Build history of the part. All positions in model axes, mm. A direction names the side the tool comes from. Coordinates: 2 decimals unless noted, no trailing zeros. One line per item, written item: value.
```python
from build123d import *

# Parameters (mm, degrees)
EXTRUDE_1_DEPTH          = 1
SKETCH_2_R               = 5
CUT_EXTRUDE_2_DEPTH      = 302.498287555
SKETCH_7_W               = 10
SKETCH_7_H               = 4
EXTRUDE_2_DEPTH          = 10
CUT_EXTRUDE_3_DEPTH      = 303.724763765
CUT_EXTRUDE_3_DEPTH_BACK = 303.724763765
SKETCH_8_R               = 3
SKETCH_9_W               = 84.692171331
SKETCH_9_H               = 26.273118844
SKETCH_9_W_2             = 56.255383877
SKETCH_9_H_2             = 8.345578926
SKETCH_9_W_3             = 22.254877138
SKETCH_9_H_3             = 20.70939956
CUT_EXTRUDE_4_DEPTH      = 302.662422914


with BuildPart() as part:
    # 草图1 → 凸台-拉伸1 (new body)
    with BuildSketch(Plane.XY):
        with BuildLine():
            add(Edge.make_bspline(
                [(0, 0), (-0.00021229, 0.506970744), (0.044864754, 1.381714413), (0.226017079, 2.650839475), (0.688025344, 4.299952552), (1.335546305, 5.873041675), (2.26695445, 7.542579189), (3.571946964, 9.346109572), (5.391381815, 11.324673938), (7.954469743, 13.539518757), (11.584975672, 16.021510412), (16.648123966, 18.726988569), (23.793189999, 21.649781435), (33.085765079, 24.436937203), (46.643058908, 27.284493785), (64.063199307, 29.362693495), (84.450847037, 30.260343335), (107.414943041, 29.859960777), (130.332556147, 28.428346139), (153.186136376, 26.214758658), (175.970846287, 23.391654718), (195.848592789, 20.487628812), (212.844945694, 17.732999103), (226.980485609, 15.27094618), (238.271313866, 13.203878393), (248.135151077, 11.310105462), (256.577305747, 9.625486685), (263.604664912, 8.179483676), (269.219788458, 6.997398786), (274.1309907, 5.93944771), (278.331979904, 5.017052178), (281.838528118, 4.234963306), (284.626645762, 3.606112196), (287.446648095, 2.96209323), (290.200347561, 2.326575377), (293.076089097, 1.653806717), (295.700233888, 1.034172197), (298.078453529, 0.464134201), (299.36547076, 0.153714708), (299.999999998, 0)],
                knots=[0, 0, 0, 0, 0, 0.005874531, 0.010168378, 0.014828146, 0.019835444, 0.025574736, 0.032308878, 0.040609511, 0.050966894, 0.064812119, 0.083253248, 0.107120705, 0.140429682, 0.177263566, 0.243881637, 0.310499708, 0.377117784, 0.443735861, 0.510353937, 0.576972013, 0.643590091, 0.67689913, 0.710208169, 0.743517207, 0.776826246, 0.793480766, 0.810135286, 0.826789806, 0.843444325, 0.851771585, 0.860098845, 0.868426105, 0.876753365, 0.885080625, 0.893407884, 0.901735144, 0.910062404, 0.910062404, 0.910062404, 0.910062404, 0.910062404], degree=4))
            add(Edge.make_bspline(
                [(0, 0), (-0.00021229, -0.506970744), (0.044864754, -1.381714413), (0.226017079, -2.650839475), (0.688025344, -4.299952552), (1.335546305, -5.873041675), (2.26695445, -7.542579189), (3.571946964, -9.346109572), (5.391381815, -11.324673938), (7.954469743, -13.539518757), (11.584975672, -16.021510412), (16.648123966, -18.726988569), (23.793189999, -21.649781435), (33.085765079, -24.436937203), (46.643058908, -27.284493785), (64.063199307, -29.362693495), (84.450847037, -30.260343335), (107.414943041, -29.859960777), (130.332556147, -28.428346139), (153.186136376, -26.214758658), (175.970846287, -23.391654718), (195.848592789, -20.487628812), (212.844945694, -17.732999103), (226.980485609, -15.27094618), (238.271313866, -13.203878393), (248.135151077, -11.310105462), (256.577305747, -9.625486685), (263.604664912, -8.179483676), (269.219788458, -6.997398786), (274.1309907, -5.93944771), (278.331979904, -5.017052178), (281.838528118, -4.234963306), (284.626645762, -3.606112196), (287.446648095, -2.96209323), (290.200347561, -2.326575377), (293.076089097, -1.653806717), (295.700233888, -1.034172197), (298.078453529, -0.464134201), (299.36547076, -0.153714708), (299.999999998, 0)],
                knots=[0, 0, 0, 0, 0, 0.005874531, 0.010168378, 0.014828146, 0.019835444, 0.025574736, 0.032308878, 0.040609511, 0.050966894, 0.064812119, 0.083253248, 0.107120705, 0.140429682, 0.177263566, 0.243881637, 0.310499708, 0.377117784, 0.443735861, 0.510353937, 0.576972013, 0.643590091, 0.67689913, 0.710208169, 0.743517207, 0.776826246, 0.793480766, 0.810135286, 0.826789806, 0.843444325, 0.851771585, 0.860098845, 0.868426105, 0.876753365, 0.885080625, 0.893407884, 0.901735144, 0.910062404, 0.910062404, 0.910062404, 0.910062404, 0.910062404], degree=4))
        make_face()
    extrude(amount=EXTRUDE_1_DEPTH)

    # 草图2 → 切除-拉伸2 (cut, through all)
    with BuildSketch(Plane.XY.offset(1)):
        with Locations((60, 0)):
            Circle(SKETCH_2_R)
        with Locations((75, 0)):
            Circle(SKETCH_2_R)
        with Locations((90, 0)):
            Circle(SKETCH_2_R)
    extrude(amount=-CUT_EXTRUDE_2_DEPTH, mode=Mode.SUBTRACT)

    # 草图7 → 凸台-拉伸2 (add)
    with BuildSketch(Plane.XY.offset(1)):
        with Locations((60, 7)):
            Rectangle(SKETCH_7_W, SKETCH_7_H)
        with Locations((60, -7)):
            Rectangle(SKETCH_7_W, SKETCH_7_H)
        with Locations((75, 7)):
            Rectangle(SKETCH_7_W, SKETCH_7_H)
        with Locations((75, -7)):
            Rectangle(SKETCH_7_W, SKETCH_7_H)
        with Locations((90, 7)):
            Rectangle(SKETCH_7_W, SKETCH_7_H)
        with Locations((90, -7)):
            Rectangle(SKETCH_7_W, SKETCH_7_H)
    extrude(amount=EXTRUDE_2_DEPTH)

    # 草图8 → 切除-拉伸3 (cut, two sides: drawn at the far end of the back side and taken through both)
    with BuildSketch(Plane.XZ.offset(9).offset(-CUT_EXTRUDE_3_DEPTH_BACK)):
        with Locations(Location((90, 6, 0), (0, 0, 270))):
            Circle(SKETCH_8_R)
        with Locations(Location((75, 6, 0), (0, 0, 270))):
            Circle(SKETCH_8_R)
        with Locations(Location((60, 6, 0), (0, 0, 270))):
            Circle(SKETCH_8_R)
    extrude(amount=CUT_EXTRUDE_3_DEPTH + CUT_EXTRUDE_3_DEPTH_BACK, mode=Mode.SUBTRACT)

    # 草图9 → 切除-拉伸4 (cut, through all)
    with BuildSketch(Plane.XY.offset(1)):
        with Locations((145.672556633, 0)):
            Rectangle(SKETCH_9_W, SKETCH_9_H)
        with Locations((227.891963838, 0)):
            Rectangle(SKETCH_9_W_2, SKETCH_9_H_2)
        with Locations((32.543597847, 0)):
            Rectangle(SKETCH_9_W_3, SKETCH_9_H_3)
    extrude(amount=-CUT_EXTRUDE_4_DEPTH, mode=Mode.SUBTRACT)


solid = part.part
```
Item 1: Cut at A-A, the plane z = 6. Give the number of separate pieces and of enclosed holes in the cut face, then the cut area to 3 significant figures.
Check result:
separate pieces: 12
enclosed holes: 0
area: 96.0 mm^2
Item 2: Pull direction Z, two halves, no side cores. Call faces 5 (the face through (72.7, -5, 3.7)), 6 (the face through (87.07, 7.03, 6.65)), 7 (the face through (119, 14, 0)): released by +Z, released by -Z, zero draft, split by the parting line, or undercut.
Check result:
face 5: zero draft
face 6: undercut
face 7: released by -Z
Item 3: Probe probe 1 along X at (y, z) = (7.7, 6); probe 2 along Z at (x, y) = (90, 6.6); probe 3 along Z at (x, y) = (68.5, 18). List the from-to ranges inside material, lowest first. Write a range as from..to.
Check result:
probe 1: x = 55..57, 63..65, 70..72, 78..80, 85..87, 93..95
probe 2: z = 0..3, 9..11
probe 3: z = 0..1
Item 4: Drop flat-ended pins along their axis: P1, Ø6, axis at x = 60, y = 0, coming from the -Z side; P2, Ø3, axis at y = -6, z = 8, coming from the -X side; P3, Ø1.5, axis at y = 11, z = 1.5, coming from the -X side; P4, Ø5, axis at x = 92, z = 5.5, coming from the +Y side. Give the stop position or say it passes through.
Check result:
P1: passes through
P2: stops at x = 55
P3: stops at x = 4.61
P4: stops at y = 9
Item 5: Tool access for faces 1 (the face through (87.7, -9, 3.7)), 2 (the face through (87.7, 5, 3.7)), 3 (the face through (72.07, 7.03, 6.65)), 4 (the face through (62.2, 9, 3.7)): list every direction of +Z, -Z, +X, -X, +Y, -Y with a clear straight run to the whole face (end or side of a thin tool).
Check result:
face 1: +Z, +X, -X, -Y
face 2: +Z, +X, -X
face 3: +Y, -Y
face 4: +Z, +X, -X, +Y
